Read the model definition and answer for the solid it produces. Units are mm, in the model's axes. Face numbers are marked on the shaded views. A direction names the side the tool comes from. Coordinates: 2 decimals unless noted, no trailing zeros. Write each loop counter-clockwise with the first axis right and the second up, starting at its lowest first coordinate (ties: lowest second). Pieces come first, ordered by that corner, then holes.
(1) Given pin 1 (8 mm diameter, centred on y = 27.5, z = 34, fed in from -X); pin 2 (3.5 mm diameter, centred on y = 6.5, z = 56, fed in from -X); pin 3 (17.5 mm diameter, centred on x = -16.5, z = 15, fed in from +Y), each flat-ended and moving along its own axis, determine where each tip first touches the part or whether it passes through.
(2) The part is cut by section D-D, the plane x = -14. Determine the outline of the cut face in (y, z), and give its area (3 significant figures).
(3) The part is cut by section A-A, the plane x = -20. State how many separate pieces and enclosed holes the cut face has, and give its area (4 significant figures).
(4) Which of the six approach directions +Z, -Z, +X, -X, +Y, -Y give full straight-line access (tool end or side, diameter ignored) to the marked faces 4, 5, 6, 7 and 8?
(5) The part is cut by section C-C, the plane z = 15. Determine the outline of the cut face in (x, y).
(6) Straight lines are drawn through the part: line 1 along Y through (x, z) = (-35, 35); line 2 along X through (y, z) = (2, 26.5); line 3 along Y through (x, z) = (-34, 16). For each, find the intervals that lie inside material, in ascending order.
(7) Determine the mould class of the marked faces 1, 2 and 3 for opening direction X: pulls with the +X half, pulls with the -X half, needs draft (parallel to the pull), parting line crosses it, or undercut.
```python
from build123d import *

# Parameters (mm, degrees)
ESQUISSE1_W              = 40
ESQUISSE1_H              = 40
BOSS_EXTRU_1_DEPTH       = 50
ESQUISSE2_R              = 5
ENL_V_MAT_EXTRU_1_DEPTH  = 41
ESQUISSE3_R              = 5
ENL_V_MAT_EXTRU_2_DEPTH  = 41
ESQUISSE4_W              = 22
ESQUISSE4_H              = 14
ENL_V_MAT_EXTRU_3_DEPTH  = 29
ESQUISSE5_W              = 14
ESQUISSE5_H              = 20
ENL_V_MAT_EXTRU_4_DEPTH  = 29
ESQUISSE6_W              = 20
ESQUISSE6_H              = 14
ENL_V_MAT_EXTRU_5_DEPTH  = 24
ESQUISSE7_W              = 14
ESQUISSE7_H              = 22
ENL_V_MAT_EXTRU_6_DEPTH  = 24
ESQUISSE10_R             = 11
ENL_V_MAT_EXTRU_9_DEPTH  = 7
ESQUISSE11_R             = 12.5
ENL_V_MAT_EXTRU_10_DEPTH = 1.5
BOSS_EXTRU_2_DEPTH       = 20
ESQUISSE14_R             = 11
ENL_V_MAT_EXTRU_11_DEPTH = 7
ESQUISSE15_R             = 12.5
ENL_V_MAT_EXTRU_12_DEPTH = 1.5


with BuildPart() as part:
    # Esquisse1 → Boss.-Extru.1 (new body)
    with BuildSketch(Plane.XY):
        with Locations((-20, 20)):
            Rectangle(ESQUISSE1_W, ESQUISSE1_H)
    extrude(amount=BOSS_EXTRU_1_DEPTH)

    # Esquisse2 → Enlèv. mat.-Extru.1 (cut, through all)
    with BuildSketch(Plane(origin=(0, 40, 0), x_dir=(1, 0, 0), z_dir=(0, 1, 0))):
        with Locations(Location((-20, -15, 0), (0, 0, 270))):  # turned: the seam where the file's is
            Circle(ESQUISSE2_R)
    extrude(amount=-ENL_V_MAT_EXTRU_1_DEPTH, mode=Mode.SUBTRACT)

    # Esquisse3 → Enlèv. mat.-Extru.2 (cut, through all)
    with BuildSketch(Plane.ZY.offset(40)):
        with Locations((35, 20)):
            Circle(ESQUISSE3_R)
    extrude(amount=-ENL_V_MAT_EXTRU_2_DEPTH, mode=Mode.SUBTRACT)

    # Esquisse4 → Enlèv. mat.-Extru.3 (cut)
    with BuildSketch(Plane.ZY.offset(40)):
        with Locations((11, 20)):
            Rectangle(ESQUISSE4_W, ESQUISSE4_H)
    extrude(amount=-ENL_V_MAT_EXTRU_3_DEPTH, mode=Mode.SUBTRACT)

    # Esquisse5 → Enlèv. mat.-Extru.4 (cut)
    with BuildSketch(Plane.XZ):
        with Locations((-20, 35)):
            Rectangle(ESQUISSE5_W, ESQUISSE5_H)
    extrude(amount=-ENL_V_MAT_EXTRU_4_DEPTH, mode=Mode.SUBTRACT)

    # Esquisse6 → Enlèv. mat.-Extru.5 (cut)
    with BuildSketch(Plane(origin=(0, 0, 0), x_dir=(0, 0, -1), z_dir=(1, 0, 0))):
        with Locations((-15, 20)):
            Rectangle(ESQUISSE6_W, ESQUISSE6_H)
    extrude(amount=-ENL_V_MAT_EXTRU_5_DEPTH, mode=Mode.SUBTRACT)

    # Esquisse7 → Enlèv. mat.-Extru.6 (cut)
    with BuildSketch(Plane(origin=(0, 40, 0), x_dir=(1, 0, 0), z_dir=(0, 1, 0))):
        with Locations((-20, -39)):
            Rectangle(ESQUISSE7_W, ESQUISSE7_H)
    extrude(amount=-ENL_V_MAT_EXTRU_6_DEPTH, mode=Mode.SUBTRACT)

    # Esquisse10 → Enlèv. mat.-Extru.9 (cut)
    with BuildSketch(Plane(origin=(0, 40, 0), x_dir=(1, 0, 0), z_dir=(0, 1, 0))):
        with Locations(Location((-20, -15, 0), (0, 0, 270))):  # turned: the seam where the file's is
            Circle(ESQUISSE10_R)
    extrude(amount=-ENL_V_MAT_EXTRU_9_DEPTH, mode=Mode.SUBTRACT)

    # Esquisse11 → Enlèv. mat.-Extru.10 (cut)
    with BuildSketch(Plane(origin=(0, 40, 0), x_dir=(1, 0, 0), z_dir=(0, 1, 0))):
        with Locations(Location((-20, -15, 0), (0, 0, 270))):  # turned: the seam where the file's is
            Circle(ESQUISSE11_R)
    extrude(amount=-ENL_V_MAT_EXTRU_10_DEPTH, mode=Mode.SUBTRACT)

    # Esquisse13 → Boss.-Extru.2 (add)
    with BuildSketch(Plane.XY.offset(50)):
        Polygon((-10, 0), (-10, 10), (0, 10), (0, 12), (-12, 12), (-12, 0), align=None)
    extrude(amount=BOSS_EXTRU_2_DEPTH)

    # Esquisse14 → Enlèv. mat.-Extru.11 (cut)
    with BuildSketch(Plane.ZY.offset(40)):
        with Locations((35, 20)):
            Circle(ESQUISSE14_R)
    extrude(amount=-ENL_V_MAT_EXTRU_11_DEPTH, mode=Mode.SUBTRACT)

    # Esquisse15 → Enlèv. mat.-Extru.12 (cut)
    with BuildSketch(Plane.ZY.offset(40)):
        with Locations((35, 20)):
            Circle(ESQUISSE15_R)
    extrude(amount=-ENL_V_MAT_EXTRU_12_DEPTH, mode=Mode.SUBTRACT)


solid = part.part
```
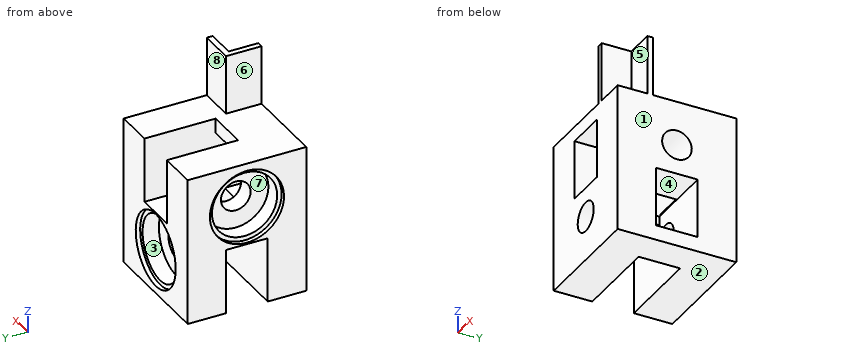
Computed:
1. pin 1: stops at x = -38.5
1. pin 2: stops at x = -12
1. pin 3: stops at y = 38.5
2. outline: (0, 0) - (13, 0) - (13, 25) - (0, 25) - close; (0, 45) - (16, 45) - (16, 50) - (0, 50) - close; (27, 0) - (40, 0) - (40, 4.03) - (38.5, 4.03) - (38.5, 5.78) - (33, 5.78) - (33, 24.22) - (38.5, 24.22) - (38.5, 25.97) - (40, 25.97) - (40, 28) - (29, 28) - (29, 25) - (27, 25) - close
2. area: 629 mm2
3. separate pieces: 5
3. enclosed holes: 0
3. area: 414.5 mm2
4. face 4: +X
4. face 5: +Z, +X, -Y
4. face 6: +Z, -X, +Y, -Y
4. face 7: -X
4. face 8: +Z, +X, -X, +Y
5. outline: (-40, 0) - (-25, 0) - (-25, 13) - (-40, 13) - close; (-40, 27) - (-25, 27) - (-25, 33) - (-31, 33) - (-31, 38.5) - (-32.5, 38.5) - (-32.5, 40) - (-40, 40) - close; (-15, 0) - (0, 0) - (0, 13) - (-15, 13) - close; (-15, 27) - (0, 27) - (0, 40) - (-7.5, 40) - (-7.5, 38.5) - (-9, 38.5) - (-9, 33) - (-15, 33) - close
6. line 1: y = 0 to 9, 31 to 40
6. line 2: x = -40 to -27, -13 to 0
6. line 3: y = 0 to 13, 27 to 40
7. face 1: pulls with the +X half
7. face 2: needs draft
7. face 3: undercut
